Can you work these out from the model? Positions are in its coordinate system, mm. Coordinates: 2 decimals unless noted, no trailing zeros. Loops run counter-clockwise (first coordinate to the right, second up) from the corner with the lowest first, then second, coordinate; pieces in that order, holes last.
```python
from build123d import *

# Parameters (mm, degrees)
SKETCH1_W           = 76.2
SKETCH1_H           = 50.8
BOSS_EXTRUDE1_DEPTH = 6.35
SKETCH3_R           = 3.96875
CUT_EXTRUDE1_DEPTH  = 92.800885072


with BuildPart() as part:
    # Sketch1 → Boss-Extrude1 (new body)
    with BuildSketch(Plane(origin=(0, 0, 0), x_dir=(1, 0, 0), z_dir=(0, 1, 0))):
        with Locations((38.1, 25.4)):
            Rectangle(SKETCH1_W, SKETCH1_H)
    extrude(amount=BOSS_EXTRUDE1_DEPTH)

    # Sketch3 → Cut-Extrude1 (cut, through all)
    with BuildSketch(Plane(origin=(0, 6.35, 0), x_dir=(1, 0, 0), z_dir=(0, 1, 0))):
        with Locations(Location((18.1, 38.1, 0), (0, 0, 270))):
            Circle(SKETCH3_R)
        with Locations(Location((18.1, 12.7, 0), (0, 0, 270))):
            Circle(SKETCH3_R)
        with Locations(Location((58.1, 38.1, 0), (0, 0, 270))):
            Circle(SKETCH3_R)
        with Locations(Location((58.1, 12.7, 0), (0, 0, 270))):
            Circle(SKETCH3_R)
    extrude(amount=-CUT_EXTRUDE1_DEPTH, mode=Mode.SUBTRACT)


solid = part.part
```
(1) I want a section at C-C on y = 1. Write out the boundary of the cut face in (x, z), then the cut area to 3 significant figures.
Check values:
outline: (0, -50.8) - (76.2, -50.8) - (76.2, 0) - (0, 0) - close; hole circle Ø7.94 at (18.1, -38.1); hole circle Ø7.94 at (18.1, -12.7); hole circle Ø7.94 at (58.1, -38.1); hole circle Ø7.94 at (58.1, -12.7)
area: 3,670 mm2
(2) If we mould it in two halves opening along Z, with no side actions, what happens to faces 1 (the flat face through (38, 3, 0)), 2 (the cylindrical face through (14.226, 3.219, -38.96)), 3 (the flat face through (38, 6.35, -26))? For each: released by +Z, released by -Z, zero draft, split by the parting line, or undercut.
Check values:
face 1: released by +Z
face 2: undercut
face 3: zero draft
(3) I want a section at A-A on x = 18.1. Write out the boundary of the cut face in (y, z), then the cut area to 3 significant figures.
Check values:
outline: (0, -50.8) - (6.35, -50.8) - (6.35, -42.07) - (0, -42.07) - close; (0, -34.13) - (6.35, -34.13) - (6.35, -16.67) - (0, -16.67) - close; (0, -8.73) - (6.35, -8.73) - (6.35, 0) - (0, 0) - close
area: 222 mm2
(4) If I drill on probe 1 along X at (y, z) = (3.75, -38.1); probe 2 along Z at (x, y) = (60, 6); probe 3 along X at (y, z) = (1, -36), over which ranges is the centre line in solid material (lowest first)?
Check values:
probe 1: x = 0 to 14.13, 22.07 to 54.13, 62.07 to 76.2
probe 2: z = -50.8 to -41.58, -34.62 to -16.18, -9.22 to 0
probe 3: x = 0 to 14.73, 21.47 to 54.73, 61.47 to 76.2
(5) I'm going to push a flat-ended pin straight in: pin 1 (5 mm diameter, centred on x = 58.1, z = -38.1, fed in from -Y). Where does the tip first touch, or does it pass through?
Check values:
pin 1: passes through
(6) I want a section at B-B on z = -38.1. Write out the boundary of the cut face in (x, y).
Check values:
outline: (0, 0) - (14.13, 0) - (14.13, 6.35) - (0, 6.35) - close; (22.07, 0) - (54.13, 0) - (54.13, 6.35) - (22.07, 6.35) - close; (62.07, 0) - (76.2, 0) - (76.2, 6.35) - (62.07, 6.35) - close
